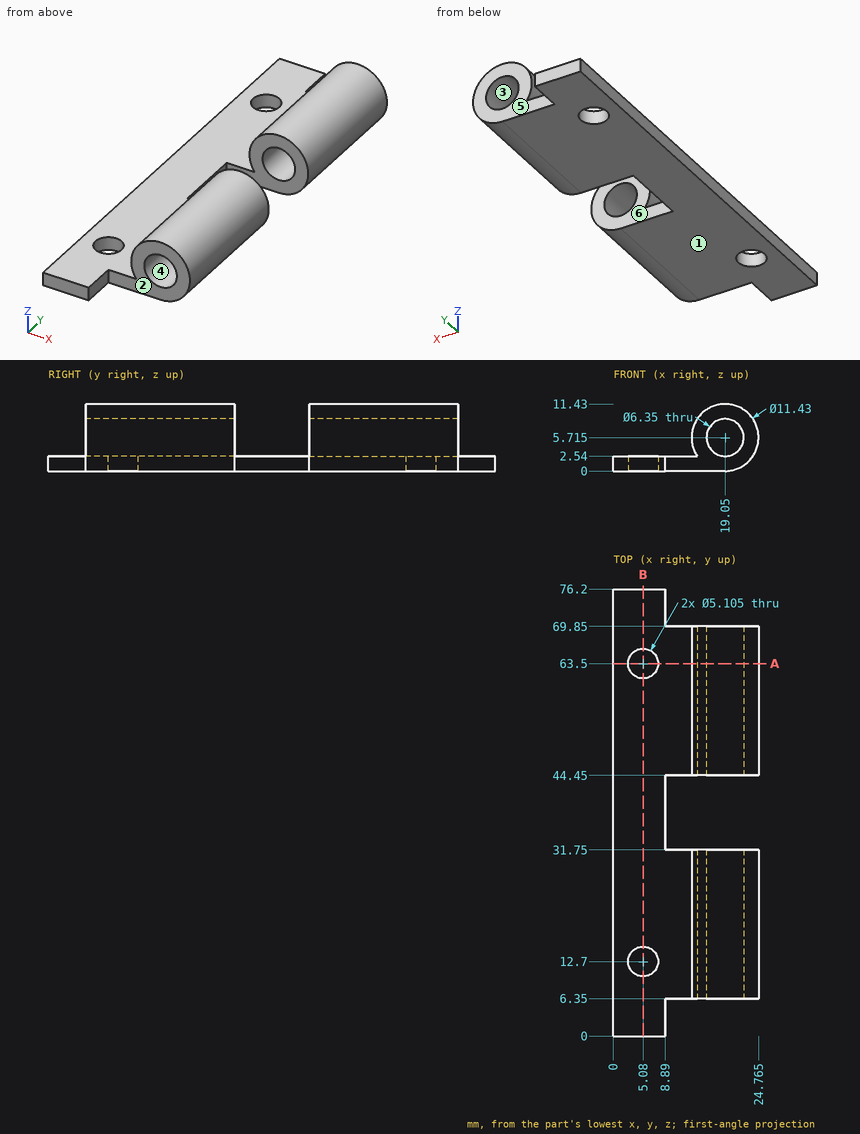
Input: dimensioned drawing with shaded views. Units: mm. Origin: part minimum x, y, z. A direction names the side the tool comes from. Coordinates: 2 decimals unless noted, no trailing zeros. Write each loop counter-clockwise with the first axis right and the second up, starting at its lowest first coordinate (ties: lowest second). Pieces come first, ordered by that corner, then holes. Notation, with made-up numbers: M 1,-3 L 54,-3 A26 cw 54,11 Z; hole C 62,34 d6. An arc over 180 degrees is marked long. Answer as a JSON object with one key per item and string values. Group by question number.
(1) Set-up query: the marked faces 5 and 6. Return all of +Z, -Z, +X, -X, +Y, -Y with unobstructed straight access to the full face (end or side cutting, diameter ignored); none if empty.
(2) Mould query, pull axis Z, two halves, no side actions, for the marked faces 1, 2, 3 and 4. Classes: pulls with the +Z half, pulls with the -Z half, needs draft (parallel to the pull), parting line crosses it, or undercut.
(3) Contact query for flat-ended pins moving along their axis: P1, Ø1.5, axis at y = 44.5, z = 2.5, coming from the +X side; P2, Ø1.3, axis at y = 72, z = 1.5, coming from the +X side; P3, Ø6, axis at x = 19, z = 7, coming from the -Y side. Output: stop coordinate, or through.
(4) Section B-B on x = 5.08. Output: boundary loops of the cut face in (y, z).
(5) Section A-A on y = 63.5. Give the number of separate pieces and of enclosed holes in the cut face.
(6) Ray query, line 1 along X through (y, z) = (30, 5.5); line 2 along Y through (x, z) = (4, 2.5); line 3 along Y through (x, z) = (5.08, 2). Return the intervals inside material, ascending. Write a range as [from, to].
Result set:
{
 "1": {"face 5": "+Z, -Z, +X, +Y", "face 6": "+Z, -Z, +X"},
 "2": {"face 1": "pulls with the -Z half", "face 2": "needs draft", "face 3": "undercut", "face 4": "undercut"},
 "3": {"P1": "stops at x = 24.21", "P2": "stops at x = 8.89", "P3": "stops at y = 6.35"},
 "4": {"outline": "M 0,0 L 10.15,0 L 10.15,2.54 L 0,2.54 Z; M 15.25,0 L 60.95,0 L 60.95,2.54 L 15.25,2.54 Z; M 66.05,0 L 76.2,0 L 76.2,2.54 L 66.05,2.54 Z"},
 "5": {"separate pieces": "2", "enclosed holes": "1"},
 "6": {"line 1": "x = [13.34, 15.88], [22.22, 24.76]", "line 2": "y = [0, 10.39], [15.01, 61.19], [65.81, 76.2]", "line 3": "y = [0, 10.15], [15.25, 60.95], [66.05, 76.2]"}
}
